```python
from build123d import *

# Parameters (mm, degrees)
ESQUISSE1_W             = 22
ESQUISSE1_H             = 10
BOSS_EXTRU_1_DEPTH      = 20
ESQUISSE2_R             = 1.5
ENL_V_MAT_EXTRU_1_DEPTH = 20
ESQUISSE4_W             = 18
ESQUISSE4_H             = 8
ENL_V_MAT_EXTRU_6_DEPTH = 18
ESQUISSE5_W             = 20
ESQUISSE5_H             = 10
BOSS_EXTRU_2_DEPTH      = 2
ESQUISSE6_W             = 8.5
ESQUISSE6_H             = 7.090406213
ENL_V_MAT_EXTRU_7_DEPTH = 8
CONG_1_R                = 5


with BuildPart() as part:
    # Esquisse1 → Boss.-Extru.1 (new body)
    with BuildSketch(Plane.XY):
        with Locations((11, 5)):
            Rectangle(ESQUISSE1_W, ESQUISSE1_H)
    extrude(amount=BOSS_EXTRU_1_DEPTH)

    # Esquisse2 → Enlèv. mat.-Extru.1 (cut)
    with BuildSketch(Plane(origin=(0, 10, 0), x_dir=(1, 0, 0), z_dir=(0, 1, 0))):
        with Locations((2, -3)):
            Circle(ESQUISSE2_R)
        with Locations((2, -17)):
            Circle(ESQUISSE2_R)
    extrude(amount=-ENL_V_MAT_EXTRU_1_DEPTH, mode=Mode.SUBTRACT)

    # Esquisse4 → Enlèv. mat.-Extru.6 (cut)
    with BuildSketch(Plane(origin=(22, 0, 0), x_dir=(0, 0, -1), z_dir=(1, 0, 0))):
        with Locations((-10, 4)):
            Rectangle(ESQUISSE4_W, ESQUISSE4_H)
    extrude(amount=-ENL_V_MAT_EXTRU_6_DEPTH, mode=Mode.SUBTRACT)

    # Esquisse5 → Boss.-Extru.2 (add)
    with BuildSketch(Plane.ZY):
        with Locations((10, 5)):
            Rectangle(ESQUISSE5_W, ESQUISSE5_H)
    extrude(amount=BOSS_EXTRU_2_DEPTH)

    # Esquisse6 → Enlèv. mat.-Extru.7 (cut)
    with BuildSketch(Plane.ZY.offset(2)):
        with Locations((10, 3.545203107)):
            Rectangle(ESQUISSE6_W, ESQUISSE6_H)
    extrude(amount=-ENL_V_MAT_EXTRU_7_DEPTH, mode=Mode.SUBTRACT)

    # Congé1
    cong_1_edges = [part.edges().sort_by_distance(p)[0] for p in [
        (4, 4, 1),
        (4, 4, 19),
    ]]
    fillet(cong_1_edges, radius=CONG_1_R)


solid = part.part
```
Input: part model. Units: mm. Frame: model coordinates. A direction names the side the tool comes from. Give positions to 0.01 mm unless a question says otherwise; leave off trailing zeros. Order: outer loops, then holes, each group sorted by start corner. A loop starts at its lowest first (then second) coordinate and runs counter-clockwise, first axis right, second up. Notation, with made-up numbers: (-2.75, -6.5) - (12.25, -6.5) arc R21 cw to (12.25, 9.5) - close; hole circle Ø2 at (16, 16). An arc over 180 degrees is marked (long way). Put each result on its own line as item: value.
Item 1: Section query A-A, the plane y = 5.5. Return loops of the section in (x, z).
Found:
outline: (-2, 0) - (22, 0) - (22, 1) - (9, 1) arc R5 cw to (4.01, 5.75) - (-2, 5.75) - close; (-2, 14.25) - (4.01, 14.25) arc R5 cw to (9, 19) - (22, 19) - (22, 20) - (-2, 20) - close; hole circle Ø3 at (2, 3); hole circle Ø3 at (2, 17)
Item 2: Section query B-B, the plane x = 2. Return loops of the section in (y, z), then the cut area to 3 significant figures.
Found:
outline: (0, 0) - (10, 0) - (10, 1.5) - (0, 1.5) - close; (0, 4.5) - (10, 4.5) - (10, 15.5) - (0, 15.5) - (0, 14.25) - (7.09, 14.25) - (7.09, 5.75) - (0, 5.75) - close; (0, 18.5) - (10, 18.5) - (10, 20) - (0, 20) - close
area: 79.7 mm^2
Item 3: Contact query for flat-ended pins moving along their axis: pin 1 (1.5 mm diameter, centred on x = 3, z = 2, fed in from -Y); pin 2 (3 mm diameter, centred on x = 0, z = 11.5, fed in from -Y); pin 3 (6 mm diameter, centred on x = 8.5, z = 9, fed in from -Y). Output: stop coordinate, or through.
Found:
pin 1: stops at y = 0
pin 2: stops at y = 7.09
pin 3: stops at y = 8
Item 4: Section query D-D, the plane x = 16. Return loops of the section in (y, z), then the cut area to 3 significant figures.
Found:
outline: (0, 0) - (10, 0) - (10, 20) - (0, 20) - (0, 19) - (8, 19) - (8, 1) - (0, 1) - close
area: 56.0 mm^2
Item 5: Section query C-C, the plane z = 3. Return loops of the section in (x, y).
Found:
outline: (-2, 0) - (0.5, 0) - (0.5, 10) - (-2, 10) - close; (3.5, 0) - (5, 0) - (5, 8) - (22, 8) - (22, 10) - (3.5, 10) - close
Item 6: Ray query, L1, parallel to Z at x = 2, y = 2.25; L2, parallel to Z at x = 12.75, y = 7; L3, parallel to Z at x = 2, y = 8. Return the intervals inside material, ascending. Write a range as from..to.
Found:
L1: z = 0..1.5, 4.5..5.75, 14.25..15.5, 18.5..20
L2: z = 0..1, 19..20
L3: z = 0..1.5, 4.5..15.5, 18.5..20
Item 7: Access query for faces 1 (the cylindrical face through (6, 4, 2)), 2 (the flat face through (1, 7.09, 10)), 3 (the cylindrical face through (0.89, 5.07, 15.99)). Directions: +Z, -Z, +X, -X, +Y, -Y. A direction counts if a zero-diameter tool reaches every point of the face in a straight line with its end or side. Return the directions, or none.
Found:
face 1: +X, -Y
face 2: +X, -X, -Y
face 3: +Y, -Y
Item 8: Draft query along Z for faces 4 (the flat face through (10, 5, 20)), 5 (the flat face through (10, 5, 0)), 6 (the flat face through (16, 4, 1)). Return one class per face: +Z half, -Z half, draft (parallel to the pull), parting line (faces both ways), or undercut.
Found:
face 4: +Z half
face 5: -Z half
face 6: undercut
